Here's how the part is built. I have some questions about the finished solid (model axes, mm). Face numbers are marked on the shaded views. A direction names the side the tool comes from. Give positions to 0.01 mm unless a question says otherwise; leave off trailing zeros. Loops run counter-clockwise (first coordinate to the right, second up) from the corner with the lowest first, then second, coordinate; pieces in that order, holes last. Notation, with made-up numbers: M 39.25,2 L 67.25,2 A19 ccw 67.25,33 Z; hole C 44,85.5 d4. An arc over 180 degrees is marked long. Answer as CSV lines item,"result". Start each with the question number.
Item 1: If we mould it in two halves opening along X, with no side actions, what happens to the marked faces 4, 5 and 6? For each: released by +X, released by -X, zero draft, split by the parting line, or undercut.
Item 2: Will these pins go through, and if not, where does the flat tip stop? P1, Ø3, axis at y = -7, z = 17, coming from the +X side; P2, Ø3.5, axis at x = 0, y = 25, coming from the +Z side; P3, Ø10, axis at y = 0, z = 48.5, coming from the -X side; P4, Ø5, axis at x = -2, z = 36.5, coming from the -Y side.
Item 3: I want a section at C-C on x = -2.5. List the corners of the cut face in (y, z) for me.
Item 4: I want a section at B-B on x = 18. List the corners of the cut face in (y, z) for me, plus the area to 3 significant figures.
Item 5: If I drill on line 1 along Y through (x, z) = (0, -3); line 2 along X through (y, z) = (18, 32); line 3 along X through (y, z) = (-25, -2.35), over which ranges is the centre line in solid material (lowest first)? Write a range as from..to.
Item 6: I want a section at D-D on z = 51.5. List the corners of the cut face in (x, y) for me, plus the area to 3 significant figures.
Item 7: I want a section at A-A on z = 11. List the corners of the cut face in (x, y) for me.
Item 8: For the marked faces 1, 2 and 3, which set-ups out of +Z, -Z, +X, -X, +Y, -Y let a thin tool reach every point of the face, with its end or its side?
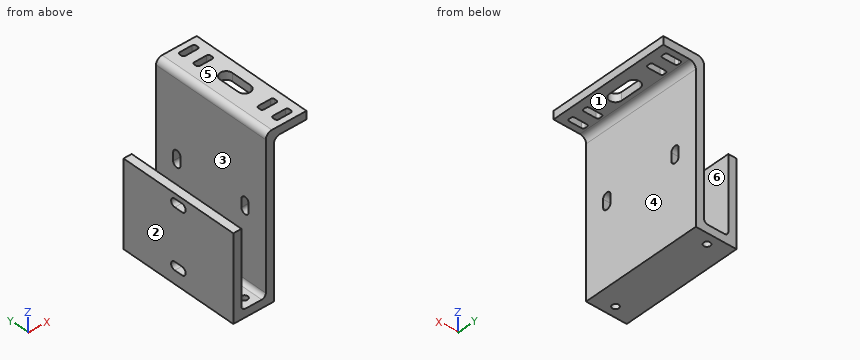
from build123d import *

# Parameters (mm, degrees)
BOSS_EXTRUDE1_DEPTH = 30
SKETCH2_W           = 8
SKETCH2_H           = 3
CUT_EXTRUDE1_DEPTH  = 86.743804441
FILLET1_R           = 1
CUT_EXTRUDE2_REACH  = 89.75
CUT_EXTRUDE3_REACH  = 86.119
SKETCH5_R           = 1.6
CUT_EXTRUDE4_DEPTH  = 86.743804441
FILLET2_R           = 2
FILLET3_R           = 3


with BuildPart() as part:
    # Sketch1 → Boss-Extrude1 (new, symmetric)
    with BuildSketch(Plane(origin=(0, 0, 0), x_dir=(1, 0, 0), z_dir=(0, 1, 0))):
        Polygon((-6, 0), (6, 0), (6, -76), (10, -76), (26, -76), (26, -72), (10, -72), (10, 4), (-10, 4), (-10, -38), (-6, -38), align=None)
    extrude(amount=BOSS_EXTRUDE1_DEPTH, both=True)

    # Sketch2 → Cut-Extrude1 (cut, through all)
    with BuildSketch(Plane(origin=(0, 0, 72), x_dir=(-1, 0, 0), z_dir=(0, 0, -1))):
        with BuildLine():
            Line((-21, -5), (-21, 5))
            ThreePointArc((-21, 5), (-18, 8), (-15, 5))
            Line((-15, 5), (-15, -5))
            ThreePointArc((-15, -5), (-18, -8), (-21, -5))
        make_face()
        with Locations((-18, 25.5)):
            Rectangle(SKETCH2_W, SKETCH2_H)
        with Locations((-18, 17.5)):
            Rectangle(SKETCH2_W, SKETCH2_H)
        with Locations((-18, -17.5)):
            Rectangle(SKETCH2_W, SKETCH2_H)
        with Locations((-18, -25.5)):
            Rectangle(SKETCH2_W, SKETCH2_H)
    extrude(amount=-CUT_EXTRUDE1_DEPTH, mode=Mode.SUBTRACT)

    # Fillet1
    fillet1_edges = [part.edges().sort_by_distance(p)[0] for p in [
        (22, 24, 74),
        (22, 27, 74),
        (14, 27, 74),
        (14, 24, 74),
        (22, 16, 74),
        (22, 19, 74),
        (14, 19, 74),
        (14, 16, 74),
        (14, -19, 74),
        (22, -19, 74),
        (22, -16, 74),
        (14, -16, 74),
        (14, -27, 74),
        (22, -27, 74),
        (22, -24, 74),
        (14, -24, 74),
    ]]
    fillet(fillet1_edges, radius=FILLET1_R)

    # Sketch3 → Cut-Extrude2 (cut, up to next)
    with BuildSketch(Plane(origin=(-6, 0, 0), x_dir=(0, 0, -1), z_dir=(1, 0, 0)), mode=Mode.PRIVATE) as cut_extrude2_sk1:
        with BuildLine():
            Line((-35.6, -2), (-35.6, 2))
            ThreePointArc((-35.6, 2), (-33.6, 4), (-31.6, 2))
            Line((-31.6, 2), (-31.6, -2))
            ThreePointArc((-31.6, -2), (-33.6, -4), (-35.6, -2))
        make_face()
    cut_extrude2_tool1 = extrude(cut_extrude2_sk1.sketch, amount=-CUT_EXTRUDE2_REACH, mode=Mode.PRIVATE) & part.part
    # Sketch3 → Cut-Extrude2 (cut, up to next)
    with BuildSketch(Plane(origin=(-6, 0, 0), x_dir=(0, 0, -1), z_dir=(1, 0, 0)), mode=Mode.PRIVATE) as cut_extrude2_sk2:
        with BuildLine():
            Line((-2.4, -2), (-2.4, 2))
            ThreePointArc((-2.4, 2), (-4.4, 4), (-6.4, 2))
            Line((-6.4, 2), (-6.4, -2))
            ThreePointArc((-6.4, -2), (-4.4, -4), (-2.4, -2))
        make_face()
    cut_extrude2_tool2 = extrude(cut_extrude2_sk2.sketch, amount=-CUT_EXTRUDE2_REACH, mode=Mode.PRIVATE) & part.part
    add(cut_extrude2_tool1.solids().sort_by_distance((-6, 0, 33.6))[0], mode=Mode.SUBTRACT)
    add(cut_extrude2_tool2.solids().sort_by_distance((-6, 0, 4.4))[0], mode=Mode.SUBTRACT)

    # Sketch4 → Cut-Extrude3 (cut, up to next)
    with BuildSketch(Plane(origin=(10, 0, 0), x_dir=(0, 0, -1), z_dir=(1, 0, 0)), mode=Mode.PRIVATE) as cut_extrude3_sk1:
        with BuildLine():
            Line((-38, 20.65), (-34, 20.65))
            ThreePointArc((-34, 20.65), (-32, 18.65), (-34, 16.65))
            Line((-34, 16.65), (-38, 16.65))
            ThreePointArc((-38, 16.65), (-40, 18.65), (-38, 20.65))
        make_face()
    cut_extrude3_tool1 = extrude(cut_extrude3_sk1.sketch, amount=-CUT_EXTRUDE3_REACH, mode=Mode.PRIVATE) & part.part
    # Sketch4 → Cut-Extrude3 (cut, up to next)
    with BuildSketch(Plane(origin=(10, 0, 0), x_dir=(0, 0, -1), z_dir=(1, 0, 0)), mode=Mode.PRIVATE) as cut_extrude3_sk2:
        with BuildLine():
            Line((-38, -20.65), (-34, -20.65))
            ThreePointArc((-34, -20.65), (-32, -18.65), (-34, -16.65))
            Line((-34, -16.65), (-38, -16.65))
            ThreePointArc((-38, -16.65), (-40, -18.65), (-38, -20.65))
        make_face()
    cut_extrude3_tool2 = extrude(cut_extrude3_sk2.sketch, amount=-CUT_EXTRUDE3_REACH, mode=Mode.PRIVATE) & part.part
    add(cut_extrude3_tool1.solids().sort_by_distance((10, 18.65, 36))[0], mode=Mode.SUBTRACT)
    add(cut_extrude3_tool2.solids().sort_by_distance((10, -18.65, 36))[0], mode=Mode.SUBTRACT)

    # Sketch5 → Cut-Extrude4 (cut, through all)
    with BuildSketch(Plane.XY):
        with Locations((0, 25)):
            Circle(SKETCH5_R)
        with Locations(Location((0, -25, 0), (0, 0, 180))):
            Circle(SKETCH5_R)
    extrude(amount=-CUT_EXTRUDE4_DEPTH, mode=Mode.SUBTRACT)

    # Fillet2
    fillet2_edges = [part.edges().sort_by_distance(p)[0] for p in [
        (6, 0, 0),
        (-6, 0, 0),
    ]]
    fillet(fillet2_edges, radius=FILLET2_R)

    # Fillet3
    fillet3_edges = [part.edges().sort_by_distance(p)[0] for p in [
        (10, 0, 72),
        (6, 0, 76),
    ]]
    fillet(fillet3_edges, radius=FILLET3_R)


solid = part.part
Result:
1,face 4,"released by +X"
1,face 5,"zero draft"
1,face 6,"undercut"
2,P1,"x = 10"
2,P2,"z = 0"
2,P3,"x = 6"
2,P4,"through"
3,outline,"M -30,-4 L 30,-4 L 30,0 L -30,0 Z"
4,outline,"M -30,72 L -27,72 L -27,76 L -30,76 Z; M -24,72 L -19,72 L -19,76 L -24,76 Z; M -16,72 L -8,72 L -8,76 L -16,76 Z; M 8,72 L 16,72 L 16,76 L 8,76 Z; M 19,72 L 24,72 L 24,76 L 19,76 Z; M 27,72 L 30,72 L 30,76 L 27,76 Z"
4,area,"128 mm^2"
5,line 1,"-30..-26.6, -23.4..23.4, 26.6..30"
5,line 2,"-10..-6, 6..10"
5,line 3,"-10..-1.6, 1.6..10"
6,outline,"M 6,-30 L 10,-30 L 10,30 L 6,30 Z"
6,area,"240 mm^2"
7,outline,"M -10,-30 L -6,-30 L -6,30 L -10,30 Z; M 6,-30 L 10,-30 L 10,30 L 6,30 Z"
8,face 1,"-Z, +X, +Y, -Y"
8,face 2,"+Z, -Z, -X, +Y, -Y"
8,face 3,"+Z, +Y, -Y"
